Geometry: see drawing. Coordinates: mm, zero at the bounding-box minimum. A direction names the side the tool comes from. Round coordinates to 2 decimals unless told otherwise and drop trailing zeros. Write each loop counter-clockwise with the first axis right and the second up, starting at its lowest first coordinate (ties: lowest second). Pieces come first, ordered by that corner, then holes. Notation, with made-up numbers: (24, 27) - (39, 27) arc R21 cw to (39, 35) - close; hole circle Ø5 at (35, 38). An arc over 180 degrees is marked (long way). One line per item, written item: value. Start each with the question number.
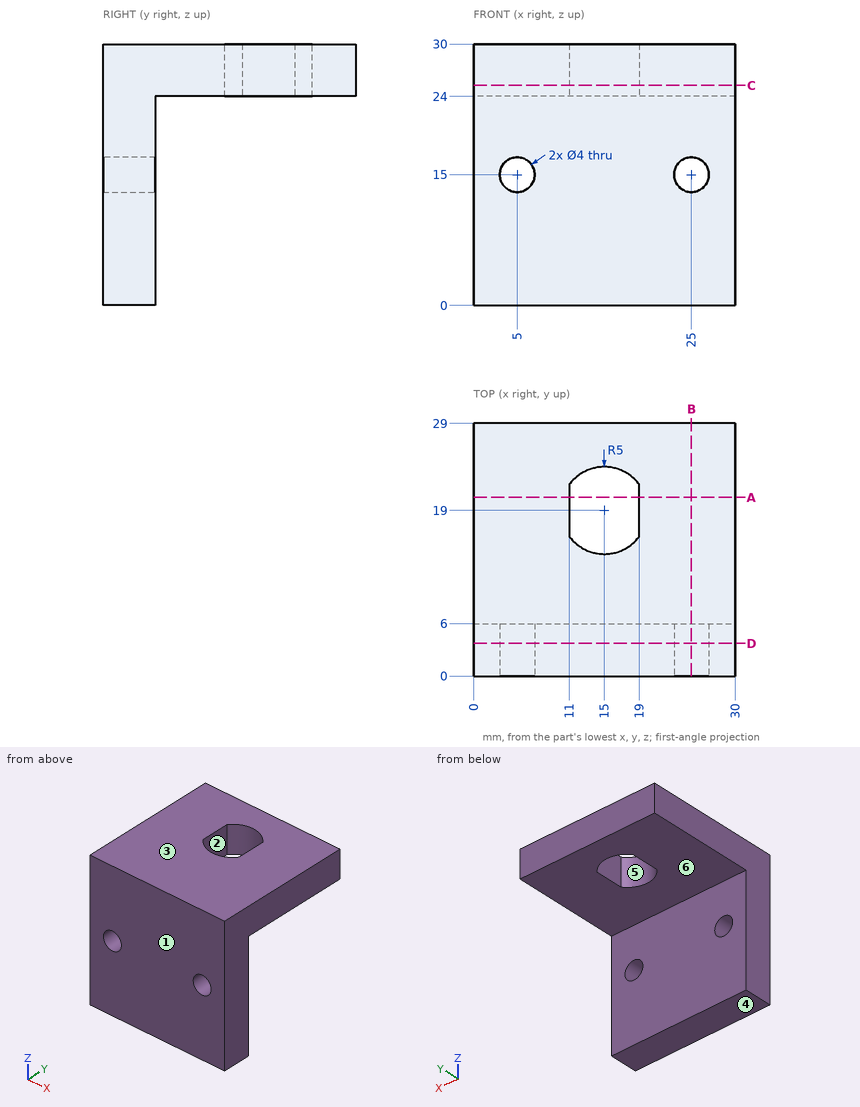
Q1. Access query for the marked faces 4, 5 and 6. Directions: +Z, -Z, +X, -X, +Y, -Y. A direction counts if a zero-diameter tool reaches every point of the face in a straight line with its end or side. Return the directions, or none.
Q2. Cut plane A-A, the plane y = 20.5. Output: boundary loops of the cut face in (x, z).
Q3. Pull-direction query (Y, two-part tool) for the marked faces 1, 2 and 3; classes: pulls with the +Y half, pulls with the -Y half, needs draft (parallel to the pull), parting line crosses it, or undercut.
Q4. Cut plane C-C, the plane z = 25.25. Output: boundary loops of the cut face in (x, y).
Q5. Cut plane D-D, the plane y = 3.75. Output: boundary loops of the cut face in (x, z).
Q6. Cut plane B-B, the plane x = 25. Output: boundary loops of the cut face in (y, z), and give its area (3 significant figures).
Q7. Material intervals for probe 1 along X at (y, z) = (3.5, 15); probe 2 along X at (y, z) = (21.5, 27.5); probe 3 along Z at (x, y) = (25, 4.6), sorted ascending. Write a range as from..to.
Q8. Contact query for a flat-ended pin moving along its axis: pin 1 Ø1.5 at (x, y) = (21.5, 22.5) entering from -Z. Output: stop coordinate, or through.
A:
1. face 4: -Z, +X, -X, +Y, -Y
1. face 5: +Z, -Z
1. face 6: -Z, +X, -X, +Y
2. outline: (0, 24) - (11, 24) - (11, 30) - (0, 30) - close; (19, 24) - (30, 24) - (30, 30) - (19, 30) - close
3. face 1: pulls with the -Y half
3. face 2: undercut
3. face 3: needs draft
4. outline: (0, 0) - (30, 0) - (30, 29) - (0, 29) - close; hole (11, 16) arc R5 ccw to (19, 16) - (19, 22) arc R5 ccw to (11, 22) - close
5. outline: (0, 0) - (30, 0) - (30, 30) - (0, 30) - close; hole circle Ø4 at (5, 15); hole circle Ø4 at (25, 15)
6. outline: (0, 0) - (6, 0) - (6, 13) - (0, 13) - close; (0, 17) - (6, 17) - (6, 24) - (29, 24) - (29, 30) - (0, 30) - close
6. area: 294 mm²
7. probe 1: x = 0..3, 7..23, 27..30
7. probe 2: x = 0..11, 19..30
7. probe 3: z = 0..13, 17..30
8. pin 1: stops at z = 24
